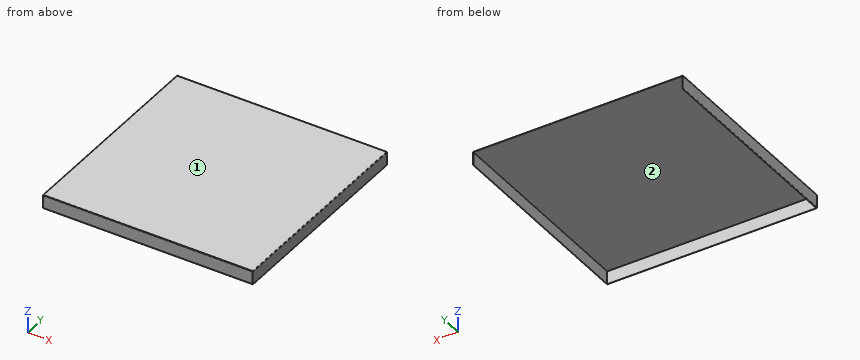
from build123d import *

# Parameters (mm, degrees)
F0_W     = 612.14
F0_H     = 612.14
F1_DEPTH = 1.5875
F3_DEPTH = 38.1
F4_R     = 1.6002
F5_R     = 1.6002
F6_R     = 1.58749
F7_R     = 1.58749


# Not quite as in the source:
# - a fillet or chamfer is up to 0.001 mm smaller than in the source, because OpenCascade refuses the exact size


with BuildPart() as f1:
    # F0 (on Top) → F1 (new body)
    with BuildSketch(Plane.XY):
        Rectangle(F0_W, F0_H)
    extrude(amount=-F1_DEPTH)

    # F2 (on face) → F3 (join)
    with BuildSketch(Plane(origin=(0, 0, -1.5875), x_dir=(1, 0, 0), z_dir=(0, 0, -1))):
        Polygon((304.4825, 304.4825), (304.4825, -306.07), (306.07, -306.07), (306.07, 306.07), (-306.07, 306.07), (-306.07, -306.07), (-304.4825, -306.07), (-304.4825, 304.4825), align=None)
    extrude(amount=F3_DEPTH)

    # F4
    f4_edges = [f1.edges().sort_by_distance(p)[0] for p in [
        (-306.07, 0, 0),
    ]]
    fillet(f4_edges, radius=F4_R)

    # F5
    f5_edges = [f1.edges().sort_by_distance(p)[0] for p in [
        (0.8001, -306.07, 0),
    ]]
    fillet(f5_edges, radius=F5_R)

    # F6 (radius 1.5875 in the source; OpenCascade refuses exactly that, so slightly less here)
    f6_edges = [f1.edges().sort_by_distance(p)[0] for p in [
        (-306.07, 0.8001, -1.6002),
        (-306.07, -304.4698, -20.64385),
        (-306.07, 306.07, -20.64385),
        (-306.07, 0.8001, -39.6875),
    ]]
    fillet(f6_edges, radius=F6_R)

    # F7 (radius 1.5875 in the source; OpenCascade refuses exactly that, so slightly less here)
    f7_edges = [f1.edges().sort_by_distance(p)[0] for p in [
        (306.07, -306.07, -19.850105),
        (306.07, -305.605035, -39.222535),
        (306.07, -305.601312, -0.468688),
        (306.07, 0.793745, -39.6875),
        (306.07, 0.006355, 0),
        (306.07, 306.07, -20.637495),
        (306.07, 305.605035, -0.464965),
    ]]
    fillet(f7_edges, radius=F7_R)


solid = f1.part
Here's how the part is built. I have some questions about the finished solid (model axes, mm). Face numbers are marked on the shaded views. Round coordinates to 2 decimals unless told otherwise and drop trailing zeros. Use CSV: the item, a comma, the result in double quotes.
1. I'm going to push a flat-ended pin straight in: P1, Ø1, axis at x = 72, y = -227, coming from the -Z side. Where does the tip first touch, or does it pass through?
Recorded:
P1,"stops at z = -1.59"
2. Thinking about a two-plate mould opening in X: for the marked faces 1 and 2, which applies, pulls with the +X half, pulls with the -X half, needs draft (parallel to the pull), parting line crosses it, or undercut?
Recorded:
face 1,"needs draft"
face 2,"undercut"
3. I need wall thicknesses on line 1 along X through (y, z) = (-79, -17.5); line 2 along Z through (x, y) = (126, 183); line 3 along Y through (x, z) = (-110.5, -20.5). Which ranges of each line are inside material? Lowest first, please.
Recorded:
line 1,"x = -306.07 to -304.48, 304.48 to 306.07"
line 2,"z = -1.59 to 0"
line 3,"y = -306.07 to -304.48"
